Geometry check sheet. Reference: the model listing, model coordinates, mm. Give positions to 0.01 mm unless a question says otherwise; leave off trailing zeros. Loops run counter-clockwise (first coordinate to the right, second up) from the corner with the lowest first, then second, coordinate; pieces in that order, holes last.
1. Material ranges on L1, parallel to X at y = 37, z = 0.3; L2, parallel to Y at x = -225.5, z = 0.6; L3, parallel to Y at x = -329, z = 1.05, recorded low to high.
2. Cross-section at A-A, the plane y = 193.5. Record the cut outline in (x, z), plus the area to 3 significant figures.
3. Cross-section at B-B, the plane z = 0.8. State how many separate pieces and enclosed holes the cut face has, plus the area to 3 significant figures.
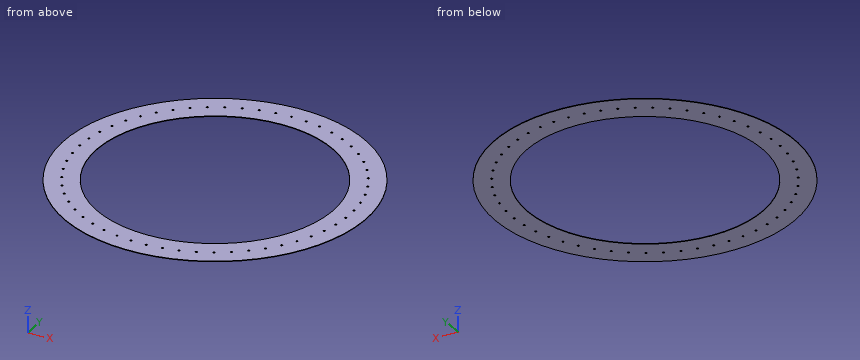
from build123d import *

# Parameters (mm, degrees)
F0_R     = 469.9
F0_R_2   = 368.3
F1_DEPTH = 1.5875
F2_R     = 3.175
F3_DEPTH = 25.4


with BuildPart() as f1:
    # F0 (on Top) → F1 (new body)
    with BuildSketch(Plane.XY):
        Circle(F0_R)
        Circle(F0_R_2, mode=Mode.SUBTRACT)
    extrude(amount=F1_DEPTH)

    # F2 (on face) → F3 (cut)
    with BuildSketch(Plane.XY.offset(1.5875)):
        with Locations((0, 419.1)):
            Circle(F2_R)
        with Locations((-47.7738, 416.368195)):
            Circle(F2_R)
        with Locations((-94.924795, 408.208394)):
            Circle(F2_R)
        with Locations((-140.838301, 394.726973)):
            Circle(F2_R)
        with Locations((-184.915764, 376.099681)):
            Circle(F2_R)
        with Locations((-226.582567, 352.569356)):
            Circle(F2_R)
        with Locations((-265.295519, 324.442749)):
            Circle(F2_R)
        with Locations((-300.549939, 292.086535)):
            Circle(F2_R)
        with Locations((-331.886231, 255.922526)):
            Circle(F2_R)
        with Locations((-358.895879, 216.422176)):
            Circle(F2_R)
        with Locations((-381.226769, 174.100432)):
            Circle(F2_R)
        with Locations((-398.587786, 129.509022)):
            Circle(F2_R)
        with Locations((-410.752601, 83.229265)):
            Circle(F2_R)
        with Locations((-417.562628, 35.864486)):
            Circle(F2_R)
        with Locations((-418.929088, -11.967841)):
            Circle(F2_R)
        with Locations((-414.834166, -59.644149)):
            Circle(F2_R)
        with Locations((-405.331247, -106.542904)):
            Circle(F2_R)
        with Locations((-390.544215, -152.052709)):
            Circle(F2_R)
        with Locations((-370.665841, -195.580275)):
            Circle(F2_R)
        with Locations((-345.955272, -236.558153)):
            Circle(F2_R)
        with Locations((-316.734647, -274.452134)):
            Circle(F2_R)
        with Locations((-283.384901, -308.768211)):
            Circle(F2_R)
        with Locations((-246.340799, -339.059022)):
            Circle(F2_R)
        with Locations((-206.085269, -364.929681)):
            Circle(F2_R)
        with Locations((-163.143102, -386.042923)):
            Circle(F2_R)
        with Locations((-118.074115, -402.123505)):
            Circle(F2_R)
        with Locations((-71.465851, -412.961793)):
            Circle(F2_R)
        with Locations((-23.925921, -418.416491)):
            Circle(F2_R)
        with Locations((23.925921, -418.416491)):
            Circle(F2_R)
        with Locations((71.465851, -412.961793)):
            Circle(F2_R)
        with Locations((118.074115, -402.123505)):
            Circle(F2_R)
        with Locations((163.143102, -386.042923)):
            Circle(F2_R)
        with Locations((206.085269, -364.929681)):
            Circle(F2_R)
        with Locations((246.340799, -339.059022)):
            Circle(F2_R)
        with Locations((283.384901, -308.768211)):
            Circle(F2_R)
        with Locations((316.734647, -274.452134)):
            Circle(F2_R)
        with Locations((345.955272, -236.558153)):
            Circle(F2_R)
        with Locations((370.665841, -195.580275)):
            Circle(F2_R)
        with Locations((390.544215, -152.052709)):
            Circle(F2_R)
        with Locations((405.331247, -106.542904)):
            Circle(F2_R)
        with Locations((414.834166, -59.644149)):
            Circle(F2_R)
        with Locations((418.929088, -11.967841)):
            Circle(F2_R)
        with Locations((417.562628, 35.864486)):
            Circle(F2_R)
        with Locations((410.752601, 83.229265)):
            Circle(F2_R)
        with Locations((398.587786, 129.509022)):
            Circle(F2_R)
        with Locations((381.226769, 174.100432)):
            Circle(F2_R)
        with Locations((358.895879, 216.422176)):
            Circle(F2_R)
        with Locations((331.886231, 255.922526)):
            Circle(F2_R)
        with Locations((300.549939, 292.086535)):
            Circle(F2_R)
        with Locations((265.295519, 324.442749)):
            Circle(F2_R)
        with Locations((226.582567, 352.569356)):
            Circle(F2_R)
        with Locations((184.915764, 376.099681)):
            Circle(F2_R)
        with Locations((140.838301, 394.726973)):
            Circle(F2_R)
        with Locations((94.924795, 408.208394)):
            Circle(F2_R)
        with Locations((47.7738, 416.368195)):
            Circle(F2_R)
    extrude(amount=-F3_DEPTH, mode=Mode.SUBTRACT)


solid = f1.part
Result:
1. L1: x = -468.44 to -420.53, -414.6 to -366.44, 366.44 to 414.6, 420.53 to 468.44
1. L2: y = -412.26 to -291.2, 291.2 to 349.58, 355.55 to 412.26
1. L3: y = -335.51 to -165.54, 165.54 to 254.6, 257.25 to 335.51
2. outline: (-428.21, 0) - (-313.37, 0) - (-313.37, 1.59) - (-428.21, 1.59) - close; (313.37, 0) - (428.21, 0) - (428.21, 1.59) - (313.37, 1.59) - close
2. area: 365 mm2
3. separate pieces: 1
3. enclosed holes: 56
3. area: 266,000 mm2
